from build123d import *

# Parameters (mm, degrees)
SKETCH1_R           = 19.5
BOSS_EXTRUDE1_DEPTH = 15
CHAMFER1_SIZE       = 5
FILLET1_R           = 3
SHELL1_T            = -3


with BuildPart() as part:
    # Sketch1 → Boss-Extrude1 (new body)
    with BuildSketch(Plane.XY):
        Circle(SKETCH1_R)
    extrude(amount=BOSS_EXTRUDE1_DEPTH)

    # Chamfer1
    chamfer1_edges = [part.edges().sort_by_distance(p)[0] for p in [
        (-19.5, 0, 15),
    ]]
    chamfer(chamfer1_edges, length=CHAMFER1_SIZE)

    # Fillet1
    fillet1_edges = [part.edges().sort_by_distance(p)[0] for p in [
        (-14.5, 0, 15),
        (-19.5, 0, 10),
    ]]
    fillet(fillet1_edges, radius=FILLET1_R)

    # Shell1
    shell1_openings = [part.faces().sort_by_distance(p)[0] for p in [
        (0, 0, 0),
    ]]
    offset(amount=SHELL1_T, openings=shell1_openings, kind=Kind.INTERSECTION)

    # Fillet2: read off the stored shape, not the designer's step
    # Fillet2 outline → Fillet2 (revolve)
    with BuildSketch(Plane.XZ):
        with BuildLine():
            Line((16.5, 9.636038969), (15.621320344, 9.636038969))
            ThreePointArc((15.621320344, 9.636038969), (16.271638598, 8.662768923), (16.5, 7.514718626))
            Line((16.5, 7.514718626), (16.5, 9.636038969))
        make_face()
        with BuildLine():
            ThreePointArc((12.014718626, 12), (13.162768923, 11.771638598), (14.136038969, 11.121320344))
            Line((14.136038969, 11.121320344), (14.136038969, 12))
            Line((14.136038969, 12), (12.014718626, 12))
        make_face()
    revolve(axis=Axis((0, 0, 0), (0, 0, 1)))


solid = part.part
Here's how the part is built. I have some questions about the finished solid (model axes, mm). Round coordinates to 2 decimals unless told otherwise and drop trailing zeros. Write each loop counter-clockwise with the first axis right and the second up, starting at its lowest first coordinate (ties: lowest second). Pieces come first, ordered by that corner, then holes.
1. I need wall thicknesses on L1, parallel to Y at x = 0, z = 4.5; L2, parallel to Z at x = -2.5, y = -12. Which ranges of each line are inside material? Lowest first, please.
2. If we mould it in two halves opening along Y, with no side actions, what happens to faces 1 (the conical face through (-3.37, -15.17, 13.96)), 2 (the cylindrical face through (15.24, -6.32, 3.7)), 3 (the flat face through (0, 0, 12)), 4 (the flat face through (-15, 9, 0))? For each: released by +Y, released by -Y, zero draft, split by the parting line, or undercut.
3. Suppose I cut it at A-A (z = 3.5). List the corners of the cut face in (x, y) for me, and give its area (3 significant figures).
4. Will these pins go through, and if not, where does the flat tip stop? pin 1 Ø1 at (y, z) = (2, 11.5) entering from +X; pin 2 Ø1 at (y, z) = (1.5, 10.5) entering from -X; pin 3 Ø8 at (x, y) = (-1, -11) entering from -Z.
Answer sheet:
1. L1: y = -19.5 to -16.5, 16.5 to 19.5
1. L2: z = 11.99 to 15
2. face 1: split by the parting line
2. face 2: undercut
2. face 3: undercut
2. face 4: zero draft
3. outline: circle Ø39 at (0, 0); hole circle Ø33 at (0, 0)
3. area: 339 mm2
4. pin 1: stops at x = 18.39
4. pin 2: stops at x = -19.18
4. pin 3: stops at z = 10.21
